Here's how the part is built. I have some questions about the finished solid (model axes, mm). Face numbers are marked on the shaded views. Round coordinates to 2 decimals unless told otherwise and drop trailing zeros. Loops run counter-clockwise (first coordinate to the right, second up) from the corner with the lowest first, then second, coordinate; pieces in that order, holes last. Notation, with made-up numbers: M 64.25,63 L 73.25,63 A4 cw 73.25,68 Z; hole C 3,-37 d2. An arc over 180 degrees is marked long. Answer as a JSON object with one key per item and string values.
from build123d import *

# Parameters (mm, degrees)
F0_R     = 1.5
F1_DEPTH = 10


# Not quite as in the source:
# - a feature names something its author has since deleted; it is built from what else it names


with BuildPart() as f1:
    # F0 (on Front) → F1 (new body, symmetric)
    with BuildSketch(Plane.XZ):
        Polygon((-5, 24), (-5, 6), (13, 6), (13, 22.4390243902), (5, 24), align=None)
        with Locations((8, 11)):
            Circle(F0_R, mode=Mode.SUBTRACT)
        with Locations((0, 19)):
            Circle(F0_R, mode=Mode.SUBTRACT)
    extrude(amount=F1_DEPTH, both=True)


solid = f1.part
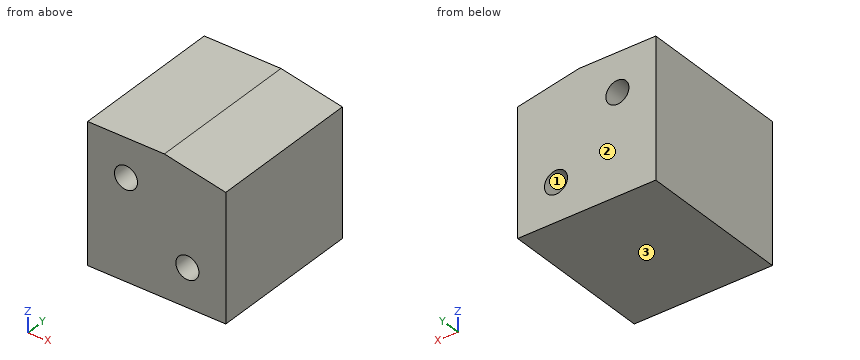
Item 1: I want a section at D-D on z = 22.75. List the corners of the cut face in (x, y) for me, plus the area to 3 significant figures.
Solution:
{"outline": "M -5,-10 L 11.41,-10 L 11.41,10 L -5,10 Z", "area": "328 mm2"}
Item 2: We'd pull the mould along Z, two halves only. Please class the marked faces 1, 2 and 3: +Z half, -Z half, draft (parallel to the pull), parting line (faces both ways), or undercut.
Solution:
{"face 1": "undercut", "face 2": "draft", "face 3": "-Z half"}
Item 3: I want a section at A-A on z = 11. List the corners of the cut face in (x, y) for me.
Solution:
{"outline": "M -5,-10 L 6.5,-10 L 6.5,10 L -5,10 Z; M 9.5,-10 L 13,-10 L 13,10 L 9.5,10 Z"}
Item 4: I want a section at C-C on y = 6. List the corners of the cut face in (x, z) for me.
Solution:
{"outline": "M -5,6 L 13,6 L 13,22.44 L 5,24 L -5,24 Z; hole C 0,19 d3; hole C 8,11 d3"}
Item 5: If I drill on L1, parallel to Z at x = 0, y = -4.5; L2, parallel to Z at x = 8.25, y = 3.5; L3, parallel to X at y = 9.25, z = 12, over which ranges is the centre line in solid material (lowest first)? Write a range as from..to.
Solution:
{"L1": "z = 6..17.5, 20.5..24", "L2": "z = 6..9.52, 12.48..23.37", "L3": "x = -5..6.88, 9.12..13"}
Item 6: For P1, Ø5, axis at x = 8, z = 11, coming from the -Y side; P2, Ø1, axis at x = 9, y = -2, coming from the +Z side, each with a flat end and sliding along its axis, tell me the tip position at first contact or that it passes through.
Solution:
{"P1": "stops at y = -10", "P2": "stops at z = 23.32"}
Item 7: I want a section at B-B on x = 8. List the corners of the cut face in (y, z) for me, plus the area to 3 significant figures.
Solution:
{"outline": "M -10,6 L 10,6 L 10,9.5 L -10,9.5 Z; M -10,12.5 L 10,12.5 L 10,23.41 L -10,23.41 Z", "area": "288 mm2"}
